```python
from build123d import *

# Parameters (mm, degrees)
AUFSATZ_LINEAR_AUSTRAGEN1_DEPTH            = 4
SCHNITT_LINEAR_AUSTRAGEN1_DEPTH            = 19.540887303
SCHNITT_LINEAR_AUSTRAGEN1_DEPTH_BACK       = 19.540887303
SKIZZE2_W                                  = 8.2
SKIZZE2_H                                  = 3
AUFSATZ_LINEAR_AUSTRAGEN2_DEPTH            = 0.6
FASE1_SIZE                                 = 0.3
FASE1_OF_SPIEGELN1_SIZE                    = 0.3
SCHNITT_LINEAR_AUSTRAGEN2_DEPTH            = 19.540887303
SCHNITT_LINEAR_AUSTRAGEN2_DEPTH_BACK       = 19.540887303
SKIZZE10_W                                 = 3.2
SKIZZE10_H                                 = 8
F_6_3_6_3_DURCHMESSER_BOHRUNG1_D           = 6.3
F_6_3_6_3_DURCHMESSER_BOHRUNG1_DEPTH       = 7.5
F_6_3_6_3_DURCHMESSER_BOHRUNG1_CSINK_D     = 7
F_6_3_6_3_DURCHMESSER_BOHRUNG1_CSINK_ANGLE = 45
F_6_3_6_3_DURCHMESSER_BOHRUNG1_TIP         = 1.89271095


with BuildPart() as part:
    # Skizze1 → Aufsatz-Linear austragen1 (new, symmetric)
    with BuildSketch(Plane(origin=(0, 0, 0), x_dir=(1, 0, 0), z_dir=(0, 1, 0))):
        with BuildLine():
            Line((2.956414504, 1.224586984), (9.656854249, 4))
            Line((9.656854249, 4), (17.656854249, 4))
            Line((17.656854249, 4), (17.656854249, -4))
            Line((17.656854249, -4), (9.656854249, -4))
            Line((9.656854249, -4), (2.956414504, -1.224586984))
            ThreePointArc((2.956414504, -1.224586984), (3.2, 0), (2.956414504, 1.224586984))
        make_face()
    extrude(amount=AUFSATZ_LINEAR_AUSTRAGEN1_DEPTH, both=True)

    # Skizze2 → Schnitt-Linear austragen1 (cut, two sides: drawn at the far end of the back side and taken through both)
    with BuildSketch(Plane.XY.offset(-SCHNITT_LINEAR_AUSTRAGEN1_DEPTH_BACK)):
        with Locations((4.1, 0)):
            Rectangle(SKIZZE2_W, SKIZZE2_H)
    extrude(amount=SCHNITT_LINEAR_AUSTRAGEN1_DEPTH + SCHNITT_LINEAR_AUSTRAGEN1_DEPTH_BACK, mode=Mode.SUBTRACT)

    # Skizze7 → Aufsatz-Linear austragen2 (add)
    with BuildSketch(Plane.XZ.offset(-1.5)):
        with BuildLine():
            Line((4.7, 0.7), (5.5, 0.7))
            ThreePointArc((5.5, 0.7), (6.2, 0), (5.5, -0.7))
            Line((5.5, -0.7), (4.7, -0.7))
            ThreePointArc((4.7, -0.7), (4, 0), (4.7, 0.7))
        make_face()
    aufsatz_linear_austragen2 = extrude(amount=AUFSATZ_LINEAR_AUSTRAGEN2_DEPTH)

    # Fase1
    fase1_edges = [part.edges().sort_by_distance(p)[0] for p in [
        (4, 0.9, 0),
        (5.1, 0.9, -0.7),
        (6.2, 0.9, 0),
        (5.1, 0.9, 0.7),
    ]]
    chamfer(fase1_edges, length=FASE1_SIZE)

    # Spiegeln1: Aufsatz-Linear austragen2 across plane
    add(aufsatz_linear_austragen2.mirror(Plane.ZX))

    # Fase1 of Spiegeln1
    fase1_of_spiegeln1_edges = [part.edges().sort_by_distance(p)[0] for p in [
        (4, -0.9, 0),
        (5.1, -0.9, -0.7),
        (6.2, -0.9, 0),
        (5.1, -0.9, 0.7),
    ]]
    chamfer(fase1_of_spiegeln1_edges, length=FASE1_OF_SPIEGELN1_SIZE)

    # Skizze10 → Schnitt-Linear austragen2 (cut, two sides: drawn at the far end of the back side and taken through both)
    with BuildSketch(Plane(origin=(0, 0, 0), x_dir=(1, 0, 0), z_dir=(0, 1, 0)).offset(-SCHNITT_LINEAR_AUSTRAGEN2_DEPTH_BACK)):
        with Locations((1.6, 0)):
            Rectangle(SKIZZE10_W, SKIZZE10_H)
    extrude(amount=SCHNITT_LINEAR_AUSTRAGEN2_DEPTH + SCHNITT_LINEAR_AUSTRAGEN2_DEPTH_BACK, mode=Mode.SUBTRACT)

    # Ø6.3 (6.3) Durchmesser Bohrung1
    with Locations(Plane(origin=(17.656854249, 0, 0), x_dir=(0, 0, -1), z_dir=(1, 0, 0))):
        with Locations((0, 0)):
            CounterSinkHole(F_6_3_6_3_DURCHMESSER_BOHRUNG1_D / 2, F_6_3_6_3_DURCHMESSER_BOHRUNG1_CSINK_D / 2, depth=F_6_3_6_3_DURCHMESSER_BOHRUNG1_DEPTH, counter_sink_angle=F_6_3_6_3_DURCHMESSER_BOHRUNG1_CSINK_ANGLE)
            with Locations((0, 0, -(F_6_3_6_3_DURCHMESSER_BOHRUNG1_DEPTH + F_6_3_6_3_DURCHMESSER_BOHRUNG1_TIP / 2))):  # 118° drill point
                Cone(0, F_6_3_6_3_DURCHMESSER_BOHRUNG1_D / 2, F_6_3_6_3_DURCHMESSER_BOHRUNG1_TIP, mode=Mode.SUBTRACT)


solid = part.part
```
Can you work these out from the model? Positions are in its coordinate system, mm. A direction names the side the tool comes from. Round coordinates to 2 decimals unless told otherwise and drop trailing zeros. Order: outer loops, then holes, each group sorted by start corner. A loop starts at its lowest first (then second) coordinate and runs counter-clockwise, first axis right, second up.
(1) We'd pull the mould along Z, two halves only. Please class faces 1 (the face through (13.438, -1.917, -2.5)), 2 (the face through (5, 0.9, 0)), 3 (the face through (6.383, 1.834, -2.644)), 4 (the face through (14, 0, 4)): +Z half, -Z half, draft (parallel to the pull), parting line (faces both ways), or undercut.
Results are:
face 1: undercut
face 2: draft
face 3: -Z half
face 4: +Z half
(2) If I drill on L1, parallel to Y at x = 14.5, z = 0; L2, parallel to Y at x = 7.5, z = 0, over which ranges is the centre line in solid material (lowest first)?
Results are:
L1: y = -4 to -3.15, 3.15 to 4
L2: y = -4 to -1.5, 1.5 to 4
(3) If we section it at A-A (x = 7.5): Please give me the cut outline in (y, z).
Results are:
outline: (-4, -3.11) - (-1.5, -3.11) - (-1.5, 3.11) - (-4, 3.11) - close; (1.5, -3.11) - (4, -3.11) - (4, 3.11) - (1.5, 3.11) - close
(4) On a 3-axis mill with a long thin cutter (end or side, diameter ignored), from which of +Z, -Z, +X, -X, +Y, -Y can I reach the whole of each face in a straight line? I mean faces 5 (the face through (5, -0.9, 0)), 6 (the face through (17.657, -0.8, -3.6)). Say none if no direction works.
Results are:
face 5: +Z, -Z, -X
face 6: +Z, -Z, +X, +Y, -Y
(5) I'm going to push a flat-ended pin straight in: pin 1 (1 mm diameter, centred on x = 6.5, y = 0, fed in from +Z). Where does the tip first touch, or does it pass through?
Results are:
pin 1: passes through
(6) If we section it at B-B (x = 11): Please give me the cut outline in (y, z).
Results are:
outline: (-4, -4) - (4, -4) - (4, 4) - (-4, 4) - close; hole circle Ø6.3 at (0, 0)
